Here's how the part is built. I have some questions about the finished solid (model axes, mm). A direction names the side the tool comes from. Coordinates: 2 decimals unless noted, no trailing zeros. Loops run counter-clockwise (first coordinate to the right, second up) from the corner with the lowest first, then second, coordinate; pieces in that order, holes last.
```python
from build123d import *

# Parameters (mm, degrees)
F2_R     = 3.8609958539
F3_DEPTH = 25
F4_R     = 2.0215779579
F5_DEPTH = 25
F6_R     = 4
F8_R     = 1
F9_SIZE  = 1


# Not quite as in the source:
# - a fillet or chamfer that OpenCascade refuses, or shapes differently, is made with other operations: its cross-section is extruded or revolved along the edge and cut away or added


with BuildPart() as f1:
    # F0 (on Front) → F1 (revolve)
    with BuildSketch(Plane.XZ):
        with BuildLine():
            Line((0, 9.6684011082), (0, 39.240504275))
            Line((0, 39.240504275), (-10, 39.240504275))
            ThreePointArc((-10, 39.240504275), (-7.7458675852, 27.3525359295), (-15, 17.6684011082))
            Line((-15, 17.6684011082), (-15, 9.6684011082))
            Line((-15, 9.6684011082), (0, 9.6684011082))
        make_face()
    revolve(axis=Axis((0, 0, 24.4544526916), (0, 0, 1)))

    # F2 (on Front) → F3 (join)
    with BuildSketch(Plane.XZ):
        with Locations((0, 29.6669229865)):
            Circle(F2_R)
    extrude(amount=F3_DEPTH)

    # F4 (on face) → F5 (join)
    with BuildSketch(Plane.XZ.offset(25)):
        with Locations((0, 29.6669229865)):
            Circle(F4_R)
    extrude(amount=F5_DEPTH)

    # F6
    f6_edges = [f1.edges().sort_by_distance(p)[0] for p in [
        (10, 0, 39.240504),
    ]]
    fillet(f6_edges, radius=F6_R)

    # F7: chamfer of 1 on 1 edges, made by hand

    # F7_s1 → F7_t2 (revolve, cut)
    with BuildSketch(Plane.XZ):
        with BuildLine():
            Line((-14.1986684737, 18.1758192127), (-15.0191266727, 16.668849252))
            Line((-15.0191266727, 16.668849252), (-15.0391266727, 16.668849252))
            ThreePointArc((-15.0391266727, 16.668849252), (-15.02, 17.1686251801), (-15.02, 17.6684011082))
            Line((-15.02, 17.6684011082), (-15.00981132, 17.685829189))
            ThreePointArc((-15.00981132, 17.685829189), (-14.6008655323, 17.9246397079), (-14.2095227335, 18.192617577))
            Line((-14.2095227335, 18.192617577), (-14.1986684737, 18.1758192127))
        make_face()
    revolve(axis=Axis((0, 0, 17.6684011082), (0, 0, 1)), mode=Mode.SUBTRACT)

    # F8
    f8_edges = [f1.edges().sort_by_distance(p)[0] for p in [
        (-3.860996, -25, 29.666923),
    ]]
    fillet(f8_edges, radius=F8_R)

    # F9
    f9_edges = [f1.edges().sort_by_distance(p)[0] for p in [
        (15, 0, 9.668401),
    ]]
    chamfer(f9_edges, length=F9_SIZE)


solid = f1.part
```
1. For pin 1 (8 mm diameter, centred on x = -10, y = -22, fed in from +Z); pin 2 (4 mm diameter, centred on x = 0.5, z = 34, fed in from -Y); pin 3 (1 mm diameter, centred on y = -8.5, z = 29, fed in from -X); pin 4 (12 mm diameter, centred on x = 7.5, y = -40.5, fed in from -Z), each with a flat end and sliding along its axis, tell me the tip position at first contact or that it passes through.
2. I want a section at B-B (y = -19). Please give me the cut outline in (x, z).
3. I want a section at A-A (z = 12). Please give me the cut outline in (x, y).
4. I need wall thicknesses on line 1 along X through (y, z) = (-8, 29.75); line 2 along Y through (x, z) = (-0.25, 11); line 3 along Z through (x, y) = (-0.25, -23.5). Which ranges of each line are inside material? Lowest first, please.
5. On a 3-axis mill with a long thin cutter (end or side, diameter ignored), from which of +Z, -Z, +X, -X, +Y, -Y can I reach the whole of each face in a straight line? I mean faces 1 (the flat face through (0, 0, 9.668)), 2 (the cylindrical face through (-3.857, -15.023, 29.837)). Say none if no direction works.
Response values:
1. pin 1: passes through
1. pin 2: stops at y = -25
1. pin 3: stops at x = -3.86
1. pin 4: stops at z = 28.31
2. outline: circle Ø7.72 at (0, 29.67)
3. outline: circle Ø30 at (0, 0)
4. line 1: x = -3.86 to 3.86
4. line 2: y = -15 to 15
4. line 3: z = 25.81 to 33.52
5. face 1: -Z, +X, -X, +Y, -Y
5. face 2: -Y
